from build123d import *

# Parameters (mm, degrees)
SKETCH1_W           = 120
SKETCH1_H           = 130
BASEMOUNT_DEPTH     = 10
SKETCH4_W           = 10
SKETCH4_H           = 10
BOSS_EXTRUDE3_DEPTH = 130
CUT_EXTRUDE2_DEPTH  = 130
SKETCH6_R           = 4
CUT_EXTRUDE3_DEPTH  = 10
SKETCH7_W           = 20
SKETCH7_H           = 20
FRONTBAR_DEPTH      = 130
SKETCH8_W           = 8
SKETCH8_H           = 8
CENTERCUT_DEPTH     = 130
SITECUTBASIC_DEPTH  = 130
SITECUTMIRROR_COUNT = 4
SKETCH11_W          = 30
SKETCH11_H          = 60
UPPERBODY_DEPTH     = 15
CUT_EXTRUDE6_START  = -10
SKETCH13_R          = 4
CUT_EXTRUDE6_DEPTH  = 10


with BuildPart() as part:
    # Sketch1 → BaseMount (new body)
    with BuildSketch(Plane(origin=(0, 0, 0), x_dir=(1, 0, 0), z_dir=(0, 1, 0))):
        Rectangle(SKETCH1_W, SKETCH1_H)
    extrude(amount=BASEMOUNT_DEPTH)


with BuildPart() as body_2:
    # Sketch4 → Boss-Extrude3 (new body)
    with BuildSketch(Plane(origin=(0, 10, 0), x_dir=(1, 0, 0), z_dir=(0, 1, 0))):
        with Locations((40, -10)):
            Rectangle(SKETCH4_W, SKETCH4_H)
    boss_extrude3 = extrude(amount=BOSS_EXTRUDE3_DEPTH)

    # Sketch5 → Cut-Extrude2 (cut)
    with BuildSketch(Plane(origin=(0, 140, 0), x_dir=(1, 0, 0), z_dir=(0, 1, 0))):
        with BuildLine():
            Line((44, -5), (42, -7))
            Line((42, -7), (40, -7))
            ThreePointArc((40, -7), (39.560660172, -5.939339828), (38.5, -5.5))
            ThreePointArc((38.5, -5.5), (38.146446609, -5.353553391), (38, -5))
            Line((38, -5), (44, -5))
        make_face()
        with BuildLine():
            Line((35, -6.975723129), (35, -5))
            Line((35, -5), (36.689326349, -5))
            ThreePointArc((36.689326349, -5), (36.32939386, -5.974805658), (35.422331587, -6.481792347))
            ThreePointArc((35.422331587, -6.481792347), (35.119977497, -6.65078791), (35, -6.975723129))
        make_face()
        Polygon((45, 3.687489646), (44.5, 4.249082756), (44.5, 5.24232749), (45, 5.687489646), align=None)
    cut_extrude2 = extrude(amount=-CUT_EXTRUDE2_DEPTH, mode=Mode.SUBTRACT)


with BuildPart() as part_1:
    add(part.part)

    add(body_2.part)  # Mirror9 merges body 2
    # Mirror9: Boss-Extrude3 across plane
    add(boss_extrude3.mirror(Plane(origin=(45, 140, 15), x_dir=(1, 0, 0), z_dir=(0, 0, -1))))

    # Mirror9 2: Cut-Extrude2 across plane
    add(cut_extrude2.mirror(Plane(origin=(45, 140, 15), x_dir=(1, 0, 0), z_dir=(0, 0, -1))), mode=Mode.SUBTRACT)

    # Sketch6 → Cut-Extrude3 (cut)
    with BuildSketch(Plane(origin=(0, 10, 0), x_dir=(1, 0, 0), z_dir=(0, 1, 0))):
        with Locations(Location((-25, -15, 0), (0, 0, 270))):
            Circle(SKETCH6_R)
        with Locations(Location((-25, 25, 0), (0, 0, 270))):
            Circle(SKETCH6_R)
    extrude(amount=-CUT_EXTRUDE3_DEPTH, mode=Mode.SUBTRACT)

    # Sketch7 → frontBar (add)
    with BuildSketch(Plane(origin=(0, 10, 0), x_dir=(1, 0, 0), z_dir=(0, 1, 0))):
        with Locations((-25, -45)):
            Rectangle(SKETCH7_W, SKETCH7_H)
    extrude(amount=FRONTBAR_DEPTH)

    # Sketch8 → centercut (cut)
    with BuildSketch(Plane(origin=(0, 140, 0), x_dir=(1, 0, 0), z_dir=(0, 1, 0))):
        with Locations((-25, -45)):
            Rectangle(SKETCH8_W, SKETCH8_H)
    extrude(amount=-CENTERCUT_DEPTH, mode=Mode.SUBTRACT)

    # Sketch10 → siteCutBasic (cut)
    with BuildSketch(Plane(origin=(0, 140, 0), x_dir=(1, 0, 0), z_dir=(0, 1, 0))):
        Polygon((-32, -53), (-29, -53), (-29, -55), (-21, -55), (-21, -53), (-18, -53), (-21, -50), (-29, -50), align=None)
    sitecutbasic = extrude(amount=-SITECUTBASIC_DEPTH, mode=Mode.SUBTRACT)

    # siteCutMirror: siteCutBasic ×4 about axis
    sitecutmirror_axis = Axis((-25, 0, 45), (0, 1, 0))
    for i in range(1, SITECUTMIRROR_COUNT):
        add(sitecutbasic.rotate(sitecutmirror_axis, i * 360 / SITECUTMIRROR_COUNT), mode=Mode.SUBTRACT)

    # Sketch11 → upperBody (add)
    with BuildSketch(Plane(origin=(0, 140, 0), x_dir=(1, 0, 0), z_dir=(0, 1, 0))):
        with Locations((-25, -30)):
            Rectangle(SKETCH11_W, SKETCH11_H)
    extrude(amount=UPPERBODY_DEPTH)

    # Sketch13 → Cut-Extrude6 (cut)
    with BuildSketch(Plane.XZ.offset(-140).offset(CUT_EXTRUDE6_START)):
        with Locations(Location((-25, 15, 0), (0, 0, 90))):
            Circle(SKETCH13_R)
    extrude(amount=CUT_EXTRUDE6_DEPTH, mode=Mode.SUBTRACT)


solid = part_1.part
Geometry check sheet. Reference: the model listing, model coordinates, mm. A direction names the side the tool comes from. Coordinates: 2 decimals unless noted, no trailing zeros. Order: outer loops, then holes, each group sorted by start corner. A loop starts at its lowest first (then second) coordinate and runs counter-clockwise, first axis right, second up. Notation, with made-up numbers: (26, -16.5) - (81, -16.5) arc R30 cw to (81, 22.5) - close; hole circle Ø7 at (-28, 33.25). An arc over 180 degrees is marked (long way). Answer in a Markdown table with one row per item. Add a question column.
1) Release check for a two-part mould opening along Z. For faces 1 (the flat face through (-25, 76, 50)), 2 (the flat face through (-25, 147, 0)), 3 (the cylindrical face through (-22.3, 5.07, 12.05)) record: +Z half, -Z half, draft (parallel to the pull), parting line (faces both ways), or undercut.
2) Material ranges on line 1 along Y through (x, z) = (-11.5, 57.5); line 2 along X through (y, z) = (13, 42); line 3 along Z through (x, y) = (-25, 145), recorded low to high. Write a range as [from, to].
3) Cross-section at C-C, the plane z = -25. Record the cut outline in (x, y).
4) Gauge pin test, flat ends, axial feed: P1, Ø4.5, axis at x = -20, y = 144, coming from the +Z side; P2, Ø1, axis at x = 37.5, y = 73.5, coming from the -Z side; P3, Ø0.6, axis at y = 104.5, z = 36, coming from the +X side. Record the tip position at first contact, or that the pin passes through.
5) Set-up check for faces 4 (the flat face through (-21, 76, 45)), 5 (the flat face through (-18, 74, 35)), 6 (the flat face through (-35, 74, 38)): record each of +Z, -Z, +X, -X, +Y, -Y from which the full face is reachable in a straight line by a thin tool's end or side.
6) Cross-section at A-A, the plane z = 15. Record the cut outline in (x, y), then the cut area to 3 significant figures.
7) Cross-section at D-D, the plane x = -49.5. Record the cut outline in (y, z), then the cut area to 3 significant figures.
8) Cross-section at B-B, the plane y = 54. State how many separate pieces and enclosed holes the cut face has, then the cut area to 3 significant figures.
Check result:
| question | item | result |
|---|---|---|
| 1 | face 1 | +Z half |
| 1 | face 2 | -Z half |
| 1 | face 3 | undercut |
| 2 | line 1 | y = [0, 10], [140, 155] |
| 2 | line 2 | x = [-30, -29], [-21, -20] |
| 2 | line 3 | z = [0, 11], [19, 60] |
| 3 | outline | (-60, 0) - (-29, 0) - (-29, 10) - (-60, 10) - close; (-21, 0) - (60, 0) - (60, 10) - (-21, 10) - close |
| 4 | P1 | stops at z = 60 |
| 4 | P2 | stops at z = 5 |
| 4 | P3 | stops at x = -15 |
| 5 | face 4 | none |
| 5 | face 5 | -Z, +X, -X |
| 5 | face 6 | +Z, -Z, -X |
| 6 | outline | (-60, 0) - (-29, 0) - (-29, 10) - (-60, 10) - close; (-40, 140) - (-29, 140) - (-29, 150) - (-21, 150) - (-21, 140) - (-10, 140) - (-10, 155) - (-40, 155) - close; (-21, 0) - (60, 0) - (60, 10) - (45, 10) - (45, 140) - (35, 140) - (35, 10) - (-21, 10) - close |
| 6 | area | 2,790 mm² |
| 7 | outline | (0, -65) - (10, -65) - (10, 65) - (0, 65) - close |
| 7 | area | 1,300 mm² |
| 8 | separate pieces | 2 |
| 8 | enclosed holes | 1 |
| 8 | area | 321 mm² |
